from build123d import *

# Parameters (mm, degrees)
F1_DEPTH      = 10
F3_DEPTH      = 7
F4_R          = 2.615
F4_W          = 5
F4_H          = 10
F5_DEPTH      = 10.001
F5_DEPTH_BACK = 25
F6_W          = 28
F6_H          = 7
F7_DEPTH      = 50
F8_W          = 28
F8_H          = 5
F9_DEPTH      = 8
F10_SIZE      = 5
F11_SIZE      = 2
F12_SIZE      = 1
F13_SIZE      = 1
F14_R         = 8
F15_SIZE      = 1
F17_DEPTH     = 10.001
F18_R         = 2
F20_DEPTH     = 7.001
F22_DEPTH     = 7
F23_R         = 8
F25_DEPTH     = 7.001
F26_SIZE      = 0.5
F27_R         = 1.99
F28_DEPTH     = 17.001
F29_R         = 2.5


# Not quite as in the source:
# - a feature names something its author has since deleted; it is built from what else it names


with BuildPart() as f1:
    # F0 (on Top) → F1 (new body)
    with BuildSketch(Plane.XY):
        Polygon((0, 14.2484272933), (-12.3395, -7.1242136467), (12.3395, -7.1242136467), align=None)
    extrude(amount=F1_DEPTH)

    # F2 (on face) → F3 (join)
    with BuildSketch(Plane(origin=(0, 0, 0), x_dir=(1, 0, 0), z_dir=(0, 0, -1))):
        Polygon((-18, 10.3923048454), (0, -20.7846096908), (18, 10.3923048454), align=None)
    extrude(amount=F3_DEPTH)

    # F4 (on Top) → F5 (cut, two sides)
    with BuildSketch(Plane.XY) as f5_sk:
        Polygon((-11.5514649078, 20.9689907423), (-11.4649338648, 8.2484272933), (13.3285973679, 8.2484272933), (13.3285973679, 20.9689907423), align=None)
        Circle(F4_R)
        with Locations((-16.5, -8)):
            Rectangle(F4_W, F4_H)
        with Locations((16.5, -8)):
            Rectangle(F4_W, F4_H)
    extrude(amount=F5_DEPTH, mode=Mode.SUBTRACT)
    extrude(f5_sk.sketch, amount=-F5_DEPTH_BACK, mode=Mode.SUBTRACT)

    # F6 (on face) → F7 (join)
    with BuildSketch(Plane.XZ.offset(10.3923048454)):
        with Locations((0, -3.5)):
            Rectangle(F6_W, F6_H)
    extrude(amount=F7_DEPTH)

    # F8 (on face) → F9 (join)
    with BuildSketch(Plane.XY):
        with Locations((0, -18.1242136467)):
            Rectangle(F8_W, F8_H)
    extrude(amount=F9_DEPTH)

    # F10
    f10_edges = [f1.edges().sort_by_distance(p)[0] for p in [
        (0, -20.624214, 0),
    ]]
    chamfer(f10_edges, length=F10_SIZE)

    # F11
    f11_edges = [f1.edges().sort_by_distance(p)[0] for p in [
        (0, -25.624214, 0),
    ]]
    chamfer(f11_edges, length=F11_SIZE)

    # F12
    f12_edges = [f1.edges().sort_by_distance(p)[0] for p in [
        (0, -27.624214, 0),
    ]]
    chamfer(f12_edges, length=F12_SIZE)

    # F13
    f13_edges = [f1.edges().sort_by_distance(p)[0] for p in [
        (0, -20.624214, 5),
    ]]
    chamfer(f13_edges, length=F13_SIZE)

    # F14
    f14_edges = [f1.edges().sort_by_distance(p)[0] for p in [
        (-14, -3.464102, -3.5),
        (14, -3.464102, -3.5),
    ]]
    fillet(f14_edges, radius=F14_R)

    # F15
    f15_edges = [f1.edges().sort_by_distance(p)[0] for p in [
        (-2.615, 0, 10),
        (-2.615, 0, -7),
    ]]
    chamfer(f15_edges, length=F15_SIZE)

    # F16 (on face) → F17 (cut, through all)
    with BuildSketch(Plane.XY):
        Polygon((12.0796923789, -6.9742136467), (-12.0796923789, -6.9742136467), (-3.2908965344, 8.2484272933), (-14, 8.2484272933), (-14, -15.7742136467), (14, -15.7742136467), (14, 8.2484272933), (7.2377682818, 8.2484272933), (3.2908965344, 8.2484272933), align=None)
    extrude(amount=F17_DEPTH, mode=Mode.SUBTRACT)

    # F18
    f18_edges = [f1.edges().sort_by_distance(p)[0] for p in [
        (-12.079692, -6.974214, 5),
        (12.079692, -6.974214, 5),
        (3.290897, 8.248427, 5),
        (-3.290897, 8.248427, 5),
        (-7.237768, 8.248427, -3.5),
        (7.237768, 8.248427, -3.5),
        (-14, -15.774214, 4),
        (14, -15.774214, 4),
    ]]
    fillet(f18_edges, radius=F18_R)

    # F19 (on face) → F20 (cut, through all)
    with BuildSketch(Plane.XY):
        with BuildLine():
            Line((6.5, -50.8923048454), (6.5, -44.3923048454))
            ThreePointArc((6.5, -44.3923048454), (0, -37.8923048454), (-6.5, -44.3923048454))
            Line((-6.5, -44.3923048454), (-6.5, -50.8923048454))
            Line((-6.5, -50.8923048454), (-6.5, -60.3923048454))
            Line((-6.5, -60.3923048454), (6.5, -60.3923048454))
            Line((6.5, -60.3923048454), (6.5, -50.8923048454))
        make_face()
    extrude(amount=-F20_DEPTH, mode=Mode.SUBTRACT)

    # F21 (on face) → F22 (join, through all)
    with BuildSketch(Plane.XY):
        Polygon((-14, -60.3923048454), (-14, -28.6242136467), (-14, -21.6960104164), (-18, -28.6242136467), (-18, -60.3923048454), align=None)
        Polygon((14, -28.6242136467), (14, -60.3923048454), (18, -60.3923048454), (18, -28.6242136467), (14, -21.6960104164), align=None)
    extrude(amount=-F22_DEPTH)

    # F23
    f23_edges = [f1.edges().sort_by_distance(p)[0] for p in [
        (18, -28.624214, -3.5),
        (14, -21.69601, -3.5),
        (-14, -21.69601, -3.5),
        (-18, -28.624214, -3.5),
        (-18, -60.392305, -3.5),
        (18, -60.392305, -3.5),
    ]]
    fillet(f23_edges, radius=F23_R)

    # F24 (on face) → F25 (cut, through all)
    with BuildSketch(Plane.XY):
        with BuildLine():
            Line((-11, -52.1423048454), (-11, -43.1423048454))
            ThreePointArc((-11, -43.1423048454), (-13, -41.1423048454), (-15, -43.1423048454))
            Line((-15, -43.1423048454), (-15, -52.1423048454))
            ThreePointArc((-15, -52.1423048454), (-13, -54.1423048454), (-11, -52.1423048454))
        make_face()
        with BuildLine():
            Line((15, -52.1423048454), (15, -43.1423048454))
            ThreePointArc((15, -43.1423048454), (13, -41.1423048454), (11, -43.1423048454))
            Line((11, -43.1423048454), (11, -52.1423048454))
            ThreePointArc((11, -52.1423048454), (13, -54.1423048454), (15, -52.1423048454))
        make_face()
    extrude(amount=-F25_DEPTH, mode=Mode.SUBTRACT)

    # F26
    f26_edges = [f1.edges().sort_by_distance(p)[0] for p in [
        (6.5, -52.392305, -7),
        (6.5, -52.392305, 0),
        (0, -6.974214, 10),
        (0, -15.774214, 8),
        (0, -37.892305, -7),
        (-6.5, -52.392305, -7),
        (-11, -47.642305, -7),
        (-13, -54.142305, -7),
        (-15, -47.642305, -7),
        (-13, -41.142305, -7),
        (15, -47.642305, -7),
        (13, -54.142305, -7),
        (11, -47.642305, -7),
        (13, -41.142305, -7),
        (-6.5, -52.392305, 0),
        (0, -37.892305, 0),
        (14, -19.199214, 8),
        (13.414214, -16.36, 8),
        (-14, -19.199214, 8),
        (-13.414214, -16.36, 8),
        (3.136196, 7.980478, 10),
        (7.107944, 1.637107, 10),
        (10.347642, -5.974214, 10),
        (0, 8.248427, 10),
        (-10.347642, -5.974214, 10),
        (-3.136196, 7.980478, 10),
        (-7.107944, 1.637107, 10),
    ]]
    chamfer(f26_edges, length=F26_SIZE)

    # F27 (on face) → F28 (cut, through all)
    with BuildSketch(Plane(origin=(0, 0, -7), x_dir=(1, 0, 0), z_dir=(0, 0, -1))):
        with Locations((-7, 9.0015727067)):
            Circle(F27_R)
        with Locations((7, 9.0015727067)):
            Circle(F27_R)
    extrude(amount=-F28_DEPTH, mode=Mode.SUBTRACT)

    # F29
    f29_edges = [f1.edges().sort_by_distance(p)[0] for p in [
        (-6.5, -60.392305, -3.5),
        (6.5, -60.392305, -3.5),
    ]]
    fillet(f29_edges, radius=F29_R)


solid = f1.part
The listing builds one solid part. Answer for the finished solid, in the listing's coordinates (mm). A direction names the side the tool comes from. Round coordinates to 2 decimals unless told otherwise and drop trailing zeros. Loops run counter-clockwise (first coordinate to the right, second up) from the corner with the lowest first, then second, coordinate; pieces in that order, holes last. Notation, with made-up numbers: M 87,12.25 L 139,12.25 A13 ccw 139,21.25 Z; hole C 69.5,80 d3. An arc over 180 degrees is marked long. Return JSON: item names as keys, results as strings.
Q1. Find section B-B, the plane y = -48. Determine the outline of the cut face in (x, z).
Results list:
{"outline": "M -18,-7 L -15.5,-7 L -15,-6.5 L -15,0 L -18,0 Z; M -11,-6.5 L -10.5,-7 L -7,-7 L -6.5,-6.5 L -6.5,-0.5 L -7,0 L -11,0 Z; M 6.5,-6.5 L 7,-7 L 10.5,-7 L 11,-6.5 L 11,0 L 7,0 L 6.5,-0.5 Z; M 15,-6.5 L 15.5,-7 L 18,-7 L 18,0 L 15,0 Z"}
Q2. Find section C-C, the plane x = 0. Determine the outline of the cut face in (y, z) (3 decimals), plus the area to 3 significant figures.
Results list:
{"outline": "M -37.892,-6.5 L -37.392,-7 L -3.615,-7 L -2.615,-6 L -2.615,9 L -3.615,10 L -6.474,10 L -6.974,9.5 L -6.974,0 L -15.774,0 L -15.774,7.5 L -16.274,8 L -20.624,8 L -20.624,6 L -21.331,4.293 L -24.21,1.414 L -26.7,0.383 L -28.624,0 L -37.392,0 L -37.892,-0.5 Z; M 2.615,-6 L 3.615,-7 L 8.248,-7 L 8.248,9.5 L 7.748,10 L 3.615,10 L 2.615,9 Z", "area": "437 mm2"}
Q3. Which of the six approach directions +Z, -Z, +X, -X, +Y, -Y give full straight-line access (tool end or side, diameter ignored) to faces 1 (the face through (-13.04, -54.14, -3.2)), 2 (the face through (14, -14, -1)), 3 (the face through (-14, -14, -1))?
Results list:
{"face 1": "+Z, -Z", "face 2": "+Z, +X, +Y", "face 3": "+Z, -X, +Y"}
Q4. Find section A-A, the plane z = 6.75. Determine the outline of the cut face in (x, y) (3 decimals).
Results list:
{"outline": "M -14,-20.624 L 14,-20.624 L 14,-17.774 A2 ccw 12,-15.774 L -12,-15.774 A2 ccw -14,-17.774 Z; M -10.348,-3.974 A2 ccw -8.616,-6.974 L 8.616,-6.974 A2 ccw 10.348,-3.974 L 3.868,7.248 A2 ccw 2.136,8.248 L -2.136,8.248 A2 ccw -3.868,7.248 Z; hole C 0,0 d5.23"}
Q5. Find the intervals of material crossed by line 1 along Y through (x, z) = (0.5, 3); line 2 along Y through (x, z) = (0, 1) (3 decimals); line 3 along X through (y, z) = (-16.5, -2.25), in increasing order. Write a range as from..to.
Results list:
{"line 1": "y = -22.62..-15.77, -6.97..-2.57, 2.57..8.25", "line 2": "y = -25.21..-15.774, -6.974..-2.615, 2.615..8.248", "line 3": "x = -14..14"}
Q6. The mould has two halves that part along X. Classify faces 4 (the face through (0, -18, 8)), 5 (the face through (7.25, -59.68, -3.55)), 6 (the face through (13.399, -16.345, 3.802)), 7 (the face through (-13.735, -3.565, -3.451)): released by +X, released by -X, zero draft, split by the parting line, or undercut.
Results list:
{"face 4": "zero draft", "face 5": "undercut", "face 6": "released by +X", "face 7": "released by -X"}
Q7. Each of these flat-tipped pins is pushed along its axis until it touches: pin 1 Ø6 at (x, z) = (-4.5, 5.5) entering from +Y; pin 2 Ø1.6 at (x, z) = (2.5, 7) entering from -Y; pin 3 Ø7.5 at (x, z) = (4, 6) entering from -Y; pin 4 Ø10 at (x, y) = (12.5, -21.5) entering from +Z. Where does it stop, or does it pass through?
Results list:
{"pin 1": "stops at y = 8.25", "pin 2": "stops at y = -20.62", "pin 3": "stops at y = -23.37", "pin 4": "stops at z = 8"}
Q8. Find section D-D, the plane y = 0. Determine the outline of the cut face in (x, z) (3 decimals).
Results list:
{"outline": "M -12,-7 L -3.615,-7 L -2.615,-6 L -2.615,9 L -3.615,10 L -7.476,10 L -8.053,9.5 L -8.053,0 L -12,0 Z; M 2.615,-6 L 3.615,-7 L 12,-7 L 12,0 L 8.053,0 L 8.053,9.5 L 7.476,10 L 3.615,10 L 2.615,9 Z"}
